Verification items for the finished model (mm, model axes). Round coordinates to 2 decimals unless told otherwise and drop trailing zeros. Loops run counter-clockwise (first coordinate to the right, second up) from the corner with the lowest first, then second, coordinate; pieces in that order, holes last. Notation, with made-up numbers: (3, 89.25) -> (48, 89.25) arc R22 cw to (48, 100.25) -> close; hole circle Ø1 at (81.25, -1). An arc over 180 degrees is marked (long way). Use a Markdown table: item, result. Add a question column.
```python
from build123d import *

# Parameters (mm, degrees)
F0_W     = 7
F0_H     = 3
F0_W_2   = 3
F0_H_2   = 10
F0_W_3   = 10
F0_W_4   = 9.5
F1_DEPTH = 1.5


with BuildPart() as f1:
    # F0 (on Top) → F1 (new body, symmetric)
    with BuildSketch(Plane.XY):
        with Locations((-63, 82.5)):
            Rectangle(F0_W, F0_H)
        Polygon((-59.5, 81), (-66.5, 81), (-66.5, 74), (-66.5, 64), (-66.5, 54), (-66.5, 44), (-66.5, 34), (-66.5, 24), (-66.5, 14), (-66.5, 4), (-66.5, 0), (0, 0), (0, 81), (-9.5, 81), (-19.5, 81), (-29.5, 81), (-39.5, 81), (-49.5, 81), align=None)
        with Locations((-68, 69)):
            Rectangle(F0_W_2, F0_H_2)
        with Locations((-44.5, 82.5)):
            Rectangle(F0_W_3, F0_H)
        with Locations((-68, 49)):
            Rectangle(F0_W_2, F0_H_2)
        with Locations((-24.5, 82.5)):
            Rectangle(F0_W_3, F0_H)
        with Locations((-68, 29)):
            Rectangle(F0_W_2, F0_H_2)
        with Locations((-4.75, 82.5)):
            Rectangle(F0_W_4, F0_H)
        with Locations((-68, 9)):
            Rectangle(F0_W_2, F0_H_2)
        Polygon((9.5, 81), (0, 81), (0, 0), (66.5, 0), (66.5, 4), (66.5, 14), (66.5, 24), (66.5, 34), (66.5, 44), (66.5, 54), (66.5, 64), (66.5, 74), (66.5, 81), (59.5, 81), (49.5, 81), (39.5, 81), (29.5, 81), (19.5, 81), align=None)
        with Locations((14.5, 82.5)):
            Rectangle(F0_W_3, F0_H)
        Polygon((0, -81), (0, 0), (-66.5, 0), (-66.5, -4), (-66.5, -14), (-66.5, -24), (-66.5, -34), (-66.5, -44), (-66.5, -54), (-66.5, -64), (-66.5, -74), (-66.5, -81), (-59.5, -81), (-49.5, -81), (-39.5, -81), (-29.5, -81), (-19.5, -81), (-9.5, -81), align=None)
        Polygon((66.5, 0), (0, 0), (0, -81), (9.5, -81), (19.5, -81), (29.5, -81), (39.5, -81), (49.5, -81), (59.5, -81), (66.5, -81), (66.5, -74), (66.5, -64), (66.5, -54), (66.5, -44), (66.5, -34), (66.5, -24), (66.5, -14), (66.5, -4), align=None)
        with Locations((-4.75, -82.5)):
            Rectangle(F0_W_4, F0_H)
        with Locations((34.5, 82.5)):
            Rectangle(F0_W_3, F0_H)
        with Locations((-68, -9)):
            Rectangle(F0_W_2, F0_H_2)
        with Locations((68, 9)):
            Rectangle(F0_W_2, F0_H_2)
        with Locations((68, -9)):
            Rectangle(F0_W_2, F0_H_2)
        with Locations((14.5, -82.5)):
            Rectangle(F0_W_3, F0_H)
        with Locations((-24.5, -82.5)):
            Rectangle(F0_W_3, F0_H)
        with Locations((54.5, 82.5)):
            Rectangle(F0_W_3, F0_H)
        with Locations((-68, -29)):
            Rectangle(F0_W_2, F0_H_2)
        with Locations((68, 29)):
            Rectangle(F0_W_2, F0_H_2)
        with Locations((68, -29)):
            Rectangle(F0_W_2, F0_H_2)
        with Locations((34.5, -82.5)):
            Rectangle(F0_W_3, F0_H)
        with Locations((-44.5, -82.5)):
            Rectangle(F0_W_3, F0_H)
        with Locations((-68, -49)):
            Rectangle(F0_W_2, F0_H_2)
        with Locations((68, 49)):
            Rectangle(F0_W_2, F0_H_2)
        with Locations((68, -49)):
            Rectangle(F0_W_2, F0_H_2)
        with Locations((54.5, -82.5)):
            Rectangle(F0_W_3, F0_H)
        with Locations((-63, -82.5)):
            Rectangle(F0_W, F0_H)
        with Locations((68, 69)):
            Rectangle(F0_W_2, F0_H_2)
        with Locations((-68, -69)):
            Rectangle(F0_W_2, F0_H_2)
        with Locations((68, -69)):
            Rectangle(F0_W_2, F0_H_2)
    extrude(amount=F1_DEPTH, both=True)


solid = f1.part
```
1) Go/stop test with flat-tipped pins: pin 1 (1.5 mm diameter, centred on y = 80, z = 0, fed in from -X); pin 2 (1.5 mm diameter, centred on x = -68.5, z = 0, fed in from +Y). Record where each tip stops, or that it passes through.
2) Thickness scan on line 1 (Y direction, x = -56, z = -0.8); line 2 (X direction, y = -57.5, z = -1.3). Record the ranges inside material, lowest first.
3) Sectioned sample at B-B on y = 56. Enter the section's corners in (x, z).
4) Sectioned sample at A-A on x = 27. Enter the section's corners in (y, z).
Geometry results:
| question | item | result |
|---|---|---|
| 1 | pin 1 | x = -66.5 |
| 1 | pin 2 | y = 74 |
| 2 | line 1 | -81 to 81 |
| 2 | line 2 | -66.5 to 66.5 |
| 3 | outline | (-66.5, -1.5) -> (66.5, -1.5) -> (66.5, 1.5) -> (-66.5, 1.5) -> close |
| 4 | outline | (-81, -1.5) -> (81, -1.5) -> (81, 1.5) -> (-81, 1.5) -> close |
